Verification items for this drawing (mm, ordinates from the low corner). Give positions to 0.01 mm unless a question says otherwise; leave off trailing zeros. Order: outer loops, then holes, each group sorted by start corner. A loop starts at its lowest first (then second) coordinate and runs counter-clockwise, first axis right, second up.
(1) Sectioned sample at A-A on y = 64. Count the separate pieces of the cut face and the enclosed holes in it, plus the area to 3 significant figures.
(2) Sectioned sample at B-B on z = 3.4. Record the cut outline in (x, y).
(3) Sectioned sample at D-D on x = 57. Record the cut outline in (y, z) (1 decimal).
(4) Scan lines: L1, parallel to X at y = 53.5, z = 3.2; L2, parallel to Y at x = 61, z = 2.7; L3, parallel to X at y = 41.5, z = 1.55. Record each from-to range of solid material in increasing order.
(5) Gauge pin test, flat end, axial feed: pin 1 (1.5 mm diameter, centred on x = 28, y = 32.5, fed in from +Z). Record the tip position at first contact, or that the pin passes through.
(6) Mould release check, pull along Y, two halves, no side actions. Record for the marked faces 1 and 2: pulls with the +Y half, pulls with the -Y half, needs draft (parallel to the pull), parting line crosses it, or undercut.
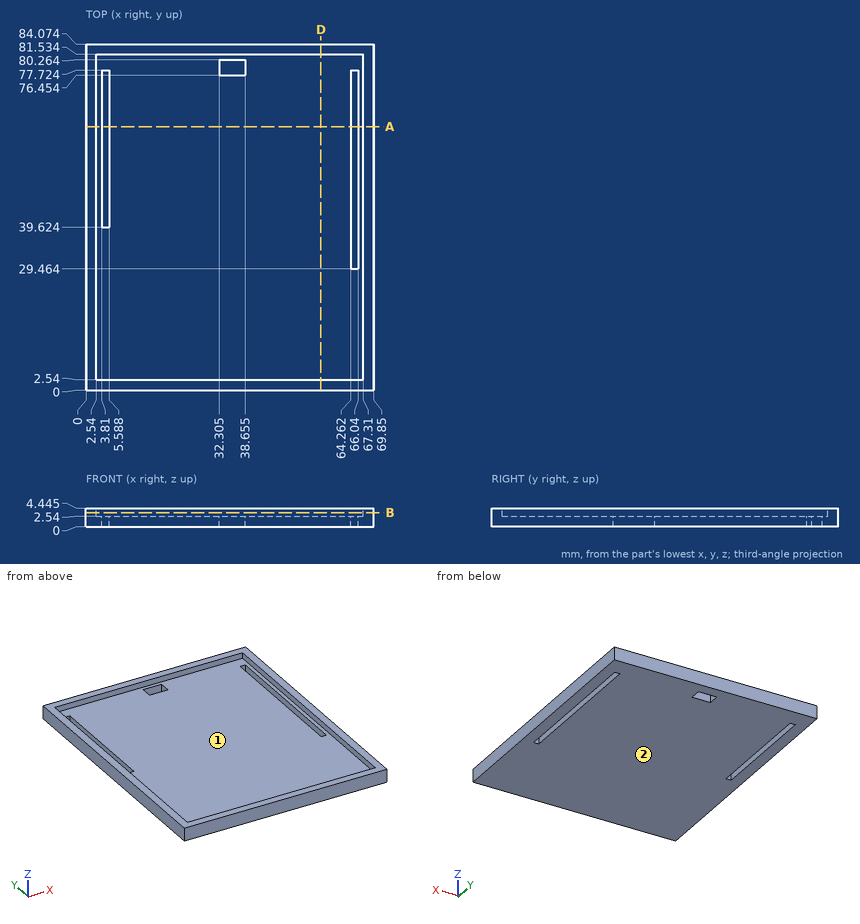
Ans:
1. separate pieces: 3
1. enclosed holes: 0
1. area: 178 mm2
2. outline: (0, 0) - (69.85, 0) - (69.85, 84.07) - (0, 84.07) - close; hole (2.54, 2.54) - (67.31, 2.54) - (67.31, 81.53) - (2.54, 81.53) - close
3. outline: (0, 0) - (84.1, 0) - (84.1, 4.4) - (81.5, 4.4) - (81.5, 2.5) - (2.5, 2.5) - (2.5, 4.4) - (0, 4.4) - close
4. L1: x = 0 to 2.54, 67.31 to 69.85
4. L2: y = 0 to 2.54, 81.53 to 84.07
4. L3: x = 0 to 3.81, 5.59 to 64.26, 66.04 to 69.85
5. pin 1: stops at z = 2.54
6. face 1: undercut
6. face 2: needs draft
